Could you check a few things on this model? Use its own coordinates, in mm. A direction names the side the tool comes from. Coordinates: 2 decimals unless noted, no trailing zeros. Loops run counter-clockwise (first coordinate to the right, second up) from the corner with the lowest first, then second, coordinate; pieces in that order, holes last.
from build123d import *

# Parameters (mm, degrees)
F0_R     = 35
F1_DEPTH = 1
F2_R     = 25
F3_DEPTH = 20
F4_R     = 4.25
F5_DEPTH = 21


with BuildPart() as f1:
    # F0 (on Top) → F1 (new body)
    with BuildSketch(Plane.XY):
        Circle(F0_R)
    extrude(amount=F1_DEPTH)

    # F2 (on face) → F3 (join)
    with BuildSketch(Plane.XY.offset(1)):
        Circle(F2_R)
    extrude(amount=F3_DEPTH)

    # F4 (on face) → F5 (cut, through all)
    with BuildSketch(Plane.XY.offset(21)):
        with BuildLine():
            ThreePointArc((-19.843134833, -2.5), (-14.1421356237, -14.1421356237), (-2.5, -19.843134833))
            Line((-2.5, -19.843134833), (-2.5, -8.6458082329))
            ThreePointArc((-2.5, -8.6458082329), (-6.3639610307, -6.3639610307), (-8.6458082329, -2.5))
            Line((-8.6458082329, -2.5), (-19.843134833, -2.5))
        make_face()
        with BuildLine():
            Line((-2.5, 8.6458082329), (-2.5, 19.843134833))
            ThreePointArc((-2.5, 19.843134833), (-14.1421356237, 14.1421356237), (-19.843134833, 2.5))
            Line((-19.843134833, 2.5), (-8.6458082329, 2.5))
            ThreePointArc((-8.6458082329, 2.5), (-6.3639610307, 6.3639610307), (-2.5, 8.6458082329))
        make_face()
        with BuildLine():
            Line((8.6458082329, 2.5), (19.843134833, 2.5))
            ThreePointArc((19.843134833, 2.5), (14.1421356237, 14.1421356237), (2.5, 19.843134833))
            Line((2.5, 19.843134833), (2.5, 8.6458082329))
            ThreePointArc((2.5, 8.6458082329), (6.3639610307, 6.3639610307), (8.6458082329, 2.5))
        make_face()
        with BuildLine():
            ThreePointArc((2.5, -19.843134833), (14.1421356237, -14.1421356237), (19.843134833, -2.5))
            Line((19.843134833, -2.5), (8.6458082329, -2.5))
            ThreePointArc((8.6458082329, -2.5), (6.3639610307, -6.3639610307), (2.5, -8.6458082329))
            Line((2.5, -8.6458082329), (2.5, -19.843134833))
        make_face()
        Circle(F4_R)
    extrude(amount=-F5_DEPTH, mode=Mode.SUBTRACT)


solid = f1.part
(1) I need wall thicknesses on probe 1 along Y at (x, z) = (0, 10.5); probe 2 along X at (y, z) = (3.5, 2); probe 3 along Y at (x, z) = (-18, 6.75). Which ranges of each line are inside material? Lowest first, please.
Answers:
probe 1: y = -25 to -4.25, 4.25 to 25
probe 2: x = -24.75 to -19.69, -8.29 to -2.41, 2.41 to 8.29, 19.69 to 24.75
probe 3: y = -17.35 to -8.72, -2.5 to 2.5, 8.72 to 17.35
(2) Which directions (+Z, -Z, +X, -X, +Y, -Y) give clear straight access to the entire face, cutting with the end or side of a thin tool? Please do faces 4 (the face through (0, -5, 21)), 5 (the face through (14, -2.5, 11)).
Answers:
face 4: +Z, +X, -X, +Y, -Y
face 5: +Z, -Z
(3) For pin 1 (5 mm diameter, centred on x = -11, z = 4.5, fed in from +Y); pin 2 (5 mm diameter, centred on y = -22, z = 5.5, fed in from -X); pin 3 (5.5 mm diameter, centred on y = -11.5, z = 6.5, fed in from +X), each with a flat end and sliding along its axis, tell me the tip position at first contact or that it passes through.
Answers:
pin 1: stops at y = 23.51
pin 2: stops at x = -15.64
pin 3: stops at x = 23.42
(4) Imagine slicing it at C-C, the plane z = 9.75. Write out the boundary of the cut face in (x, y).
Answers:
outline: circle Ø50 at (0, 0); hole (-19.84, -2.5) arc R20 ccw to (-2.5, -19.84) - (-2.5, -8.65) arc R9 cw to (-8.65, -2.5) - close; hole (-19.84, 2.5) - (-8.65, 2.5) arc R9 cw to (-2.5, 8.65) - (-2.5, 19.84) arc R20 ccw to start; hole circle Ø8.5 at (0, 0); hole (2.5, -19.84) arc R20 ccw to (19.84, -2.5) - (8.65, -2.5) arc R9 cw to (2.5, -8.65) - close; hole (2.5, 8.65) arc R9 cw to (8.65, 2.5) - (19.84, 2.5) arc R20 ccw to (2.5, 19.84) - close
(5) We'd pull the mould along Y, two halves only. Please class faces 1 (the face through (23.846, 7.509, 10.86)), 2 (the face through (-24, 8, 1)), 3 (the face through (2.5, 14, 11)): +Y half, -Y half, draft (parallel to the pull), parting line (faces both ways), or undercut.
Answers:
face 1: parting line
face 2: draft
face 3: undercut
(6) Imagine slicing it at D-D, the plane y = -22. Write out the boundary of the cut face in (x, z), and give its area (3 significant figures).
Answers:
outline: (-27.22, 0) - (27.22, 0) - (27.22, 1) - (11.87, 1) - (11.87, 21) - (-11.87, 21) - (-11.87, 1) - (-27.22, 1) - close
area: 529 mm2
(7) Imagine slicing it at A-A, the plane y = 0. Write out the boundary of the cut face in (x, z).
Answers:
outline: (-35, 0) - (-4.25, 0) - (-4.25, 21) - (-25, 21) - (-25, 1) - (-35, 1) - close; (4.25, 0) - (35, 0) - (35, 1) - (25, 1) - (25, 21) - (4.25, 21) - close
